```python
from build123d import *

# Parameters (mm, degrees)
ESKIZ_KONTUR_W        = 10.2
ESKIZ_KONTUR_H        = 3.2
PLASTINA_DEPTH        = 3
OTVERSTIYA_DEPTH      = 26.787593916
OTVERSTIYA_DEPTH_BACK = 26.787593916
ESKIZ_OTVERSTIYA_R    = 1.65
ESKIZ_OTVERSTIYA_R_2  = 0.75
ESKIZ_OTVERSTIYA_R_3  = 3


with BuildPart() as part:
    # Eskiz_kontur → Plastina (new body)
    with BuildSketch(Plane.XY):
        with BuildLine():
            Line((-20, -12), (-20, 6))
            ThreePointArc((-20, 6), (-18.828427125, 8.828427125), (-16, 10))
            Line((-16, 10), (16, 10))
            ThreePointArc((16, 10), (18.828427125, 8.828427125), (20, 6))
            Line((20, 6), (20, -12))
            ThreePointArc((20, -12), (18.828427125, -14.828427125), (16, -16))
            Line((16, -16), (-16, -16))
            ThreePointArc((-16, -16), (-18.828427125, -14.828427125), (-20, -12))
        make_face()
        with Locations((-11, -11)):
            Rectangle(ESKIZ_KONTUR_W, ESKIZ_KONTUR_H, mode=Mode.SUBTRACT)
        with Locations((11, -11)):
            Rectangle(ESKIZ_KONTUR_W, ESKIZ_KONTUR_H, mode=Mode.SUBTRACT)
    extrude(amount=PLASTINA_DEPTH)

    # Eskiz_otverstiya → Otverstiya (cut, two sides: drawn at the far end of the back side and taken through both)
    with BuildSketch(Plane.XY.offset(-OTVERSTIYA_DEPTH_BACK)):
        with Locations((0, -11)):
            Circle(ESKIZ_OTVERSTIYA_R)
        with Locations((-13, 0)):
            Circle(ESKIZ_OTVERSTIYA_R_2)
        with Locations((-11, 0)):
            Circle(ESKIZ_OTVERSTIYA_R_2)
        with Locations((-9, 0)):
            Circle(ESKIZ_OTVERSTIYA_R_2)
        with Locations((-7, 0)):
            Circle(ESKIZ_OTVERSTIYA_R_2)
        Circle(ESKIZ_OTVERSTIYA_R_3)
        with Locations((7, 0)):
            Circle(ESKIZ_OTVERSTIYA_R_2)
        with Locations((9, 0)):
            Circle(ESKIZ_OTVERSTIYA_R_2)
        with Locations((11, 0)):
            Circle(ESKIZ_OTVERSTIYA_R_2)
        with Locations((13, 0)):
            Circle(ESKIZ_OTVERSTIYA_R_2)
        with Locations((0, 7)):
            Circle(ESKIZ_OTVERSTIYA_R_2)
        with Locations((0, 9)):
            Circle(ESKIZ_OTVERSTIYA_R_2)
    extrude(amount=OTVERSTIYA_DEPTH + OTVERSTIYA_DEPTH_BACK, mode=Mode.SUBTRACT)


solid = part.part
```
Read the model definition and answer for the solid it produces. Units are mm, in the model's axes. A direction names the side the tool comes from. Coordinates: 2 decimals unless noted, no trailing zeros. Write each loop counter-clockwise with the first axis right and the second up, starting at its lowest first coordinate (ties: lowest second). Pieces come first, ordered by that corner, then holes. Notation, with made-up numbers: (-23, 52.25) - (-3, 52.25) arc R20 ccw to (-3, 76.25) - close; hole circle Ø4 at (-15, 69). An arc over 180 degrees is marked (long way). Answer as a JSON object with one key per item and string values. Group by question number.
1. A cutting plane is placed at D-D (z = 0.7). Give the number of separate pieces and of enclosed holes in the cut face, plus the area to 3 significant figures.
2. Each of these flat-tipped pins is pushed along its axis until it touches: P1, Ø1.2, axis at x = 11, y = 0, coming from the +Z side; P2, Ø8, axis at x = -7, y = 3.5, coming from the -Z side. Where does it stop, or does it pass through?
3. A cutting plane is placed at C-C (x = 0). Determine the outline of the cut face in (y, z).
4. A cutting plane is placed at A-A (x = 7). Determine the outline of the cut face in (y, z).
5. Which of the six approach directions +Z, -Z, +X, -X, +Y, -Y give full straight-line access (tool end or side, diameter ignored) to faces 1 (the cylindrical face through (-18.797, -14.859, 1.479)), 2 (the flat face through (5.9, -11, 1))?
6. A cutting plane is placed at B-B (y = 9). Determine the outline of the cut face in (x, z).
7. Consider L1, parallel to Y at x = 0, z = 2.4; L2, parallel to Y at x = 9, z = 1.25; L3, parallel to Y at x = -13.5, z = 1.2. Determine where each line is inside the solid, lowest interval first. Write a range as [from, to].
8. The mould has two halves that part along X. Classify faces 3 (the flat face through (16.1, -11, 1)), 4 (the flat face through (20, -3, 1)), 5 (the flat face through (0, -16, 1)), 6 (the flat face through (-20, -3, 1)): +X half, -X half, draft (parallel to the pull), parting line (faces both ways), or undercut.
Worked out:
{
 "1": {"separate pieces": "1", "enclosed holes": "14", "area": "906 mm²"},
 "2": {"P1": "passes through", "P2": "stops at z = 0"},
 "3": {"outline": "(-16, 0) - (-12.65, 0) - (-12.65, 3) - (-16, 3) - close; (-9.35, 0) - (-3, 0) - (-3, 3) - (-9.35, 3) - close; (3, 0) - (6.25, 0) - (6.25, 3) - (3, 3) - close; (7.75, 0) - (8.25, 0) - (8.25, 3) - (7.75, 3) - close; (9.75, 0) - (10, 0) - (10, 3) - (9.75, 3) - close"},
 "4": {"outline": "(-16, 0) - (-12.6, 0) - (-12.6, 3) - (-16, 3) - close; (-9.4, 0) - (-0.75, 0) - (-0.75, 3) - (-9.4, 3) - close; (0.75, 0) - (10, 0) - (10, 3) - (0.75, 3) - close"},
 "5": {"face 1": "+Z, -Z, -X, -Y", "face 2": "+Z, -Z"},
 "6": {"outline": "(-18.65, 0) - (-0.75, 0) - (-0.75, 3) - (-18.65, 3) - close; (0.75, 0) - (18.65, 0) - (18.65, 3) - (0.75, 3) - close"},
 "7": {"L1": "y = [-16, -12.65], [-9.35, -3], [3, 6.25], [7.75, 8.25], [9.75, 10]", "L2": "y = [-16, -12.6], [-9.4, -0.75], [0.75, 10]", "L3": "y = [-16, -12.6], [-9.4, -0.56], [0.56, 10]"},
 "8": {"face 3": "undercut", "face 4": "+X half", "face 5": "draft", "face 6": "-X half"}
}
